Geometry check sheet. Reference: the model listing, model coordinates, mm. A direction names the side the tool comes from. Coordinates: 2 decimals unless noted, no trailing zeros. Loops run counter-clockwise (first coordinate to the right, second up) from the corner with the lowest first, then second, coordinate; pieces in that order, holes last. Notation, with made-up numbers: (77, 78) - (94, 78) arc R19 cw to (94, 82) - close; hole circle Ø7 at (33, 26). An arc over 180 degrees is marked (long way). Write item = value, one per line. Start each with the question number.
from build123d import *

# Parameters (mm, degrees)
SKETCH1_R           = 3.2639
BOSS_EXTRUDE1_DEPTH = 152.4


with BuildPart() as part:
    # Sketch1 → Boss-Extrude1 (new, symmetric)
    with BuildSketch(Plane.XY):
        with BuildLine():
            Line((-6.731, 4.575738531), (-6.731, -4.575738531))
            Line((-6.731, -4.575738531), (-12.442261469, -10.287))
            Line((-12.442261469, -10.287), (-15.6718, -10.287))
            Line((-15.6718, -10.287), (-15.6718, -6.858))
            Line((-15.6718, -6.858), (-14.478, -6.858))
            Line((-14.478, -6.858), (-14.478, -4.064))
            Line((-14.478, -4.064), (-19.05, -4.064))
            Line((-19.05, -4.064), (-19.05, -15.875))
            ThreePointArc((-19.05, -15.875), (-18.12006403, -18.12006403), (-15.875, -19.05))
            Line((-15.875, -19.05), (-4.064, -19.05))
            Line((-4.064, -19.05), (-4.064, -14.478))
            Line((-4.064, -14.478), (-6.858, -14.478))
            Line((-6.858, -14.478), (-6.858, -15.6718))
            Line((-6.858, -15.6718), (-10.287, -15.6718))
            Line((-10.287, -15.6718), (-10.287, -12.442261469))
            Line((-10.287, -12.442261469), (-4.575738531, -6.731))
            Line((-4.575738531, -6.731), (4.575738531, -6.731))
            Line((4.575738531, -6.731), (10.287, -12.442261469))
            Line((10.287, -12.442261469), (10.287, -15.6718))
            Line((10.287, -15.6718), (6.858, -15.6718))
            Line((6.858, -15.6718), (6.858, -14.478))
            Line((6.858, -14.478), (4.064, -14.478))
            Line((4.064, -14.478), (4.064, -19.05))
            Line((4.064, -19.05), (15.875, -19.05))
            ThreePointArc((15.875, -19.05), (18.12006403, -18.12006403), (19.05, -15.875))
            Line((19.05, -15.875), (19.05, -4.064))
            Line((19.05, -4.064), (14.478, -4.064))
            Line((14.478, -4.064), (14.478, -6.858))
            Line((14.478, -6.858), (15.6718, -6.858))
            Line((15.6718, -6.858), (15.6718, -10.287))
            Line((15.6718, -10.287), (12.442261469, -10.287))
            Line((12.442261469, -10.287), (6.731, -4.575738531))
            Line((6.731, -4.575738531), (6.731, 4.575738531))
            Line((6.731, 4.575738531), (12.442261469, 10.287))
            Line((12.442261469, 10.287), (15.6718, 10.287))
            Line((15.6718, 10.287), (15.6718, 6.858))
            Line((15.6718, 6.858), (14.478, 6.858))
            Line((14.478, 6.858), (14.478, 4.064))
            Line((14.478, 4.064), (19.05, 4.064))
            Line((19.05, 4.064), (19.05, 15.875))
            ThreePointArc((19.05, 15.875), (18.12006403, 18.12006403), (15.875, 19.05))
            Line((15.875, 19.05), (4.064, 19.05))
            Line((4.064, 19.05), (4.064, 14.478))
            Line((4.064, 14.478), (6.858, 14.478))
            Line((6.858, 14.478), (6.858, 15.6718))
            Line((6.858, 15.6718), (10.287, 15.6718))
            Line((10.287, 15.6718), (10.287, 12.442261469))
            Line((10.287, 12.442261469), (4.575738531, 6.731))
            Line((4.575738531, 6.731), (-4.575738531, 6.731))
            Line((-4.575738531, 6.731), (-10.287, 12.442261469))
            Line((-10.287, 12.442261469), (-10.287, 15.6718))
            Line((-10.287, 15.6718), (-6.858, 15.6718))
            Line((-6.858, 15.6718), (-6.858, 14.478))
            Line((-6.858, 14.478), (-4.064, 14.478))
            Line((-4.064, 14.478), (-4.064, 19.05))
            Line((-4.064, 19.05), (-15.875, 19.05))
            ThreePointArc((-15.875, 19.05), (-18.12006403, 18.12006403), (-19.05, 15.875))
            Line((-19.05, 15.875), (-19.05, 4.064))
            Line((-19.05, 4.064), (-14.478, 4.064))
            Line((-14.478, 4.064), (-14.478, 6.858))
            Line((-14.478, 6.858), (-15.6718, 6.858))
            Line((-15.6718, 6.858), (-15.6718, 10.287))
            Line((-15.6718, 10.287), (-12.442261469, 10.287))
            Line((-12.442261469, 10.287), (-6.731, 4.575738531))
        make_face()
        with Locations(Location((0, 0, 0), (0, 0, 180))):
            Circle(SKETCH1_R, mode=Mode.SUBTRACT)
        with BuildLine():
            Line((-11.8872, 17.272), (-14.478, 17.272))
            ThreePointArc((-14.478, 17.272), (-16.453656347, 16.453656347), (-17.272, 14.478))
            Line((-17.272, 14.478), (-17.272, 11.8872))
            Line((-17.272, 11.8872), (-11.8872, 11.8872))
            Line((-11.8872, 11.8872), (-11.8872, 17.272))
        make_face(mode=Mode.SUBTRACT)
        with BuildLine():
            Line((14.478, 17.272), (11.8872, 17.272))
            Line((11.8872, 17.272), (11.8872, 11.8872))
            Line((11.8872, 11.8872), (17.272, 11.8872))
            Line((17.272, 11.8872), (17.272, 14.478))
            ThreePointArc((17.272, 14.478), (16.453656347, 16.453656347), (14.478, 17.272))
        make_face(mode=Mode.SUBTRACT)
        with BuildLine():
            Line((11.8872, -17.272), (14.478, -17.272))
            ThreePointArc((14.478, -17.272), (16.453656347, -16.453656347), (17.272, -14.478))
            Line((17.272, -14.478), (17.272, -11.8872))
            Line((17.272, -11.8872), (11.8872, -11.8872))
            Line((11.8872, -11.8872), (11.8872, -17.272))
        make_face(mode=Mode.SUBTRACT)
        with BuildLine():
            Line((-14.478, -17.272), (-11.8872, -17.272))
            Line((-11.8872, -17.272), (-11.8872, -11.8872))
            Line((-11.8872, -11.8872), (-17.272, -11.8872))
            Line((-17.272, -11.8872), (-17.272, -14.478))
            ThreePointArc((-17.272, -14.478), (-16.453656347, -16.453656347), (-14.478, -17.272))
        make_face(mode=Mode.SUBTRACT)
    extrude(amount=BOSS_EXTRUDE1_DEPTH, both=True)


solid = part.part
(1) Tool access check on faces 4 (the face through (15, 11.887, -2)), 5 (the face through (-19.05, -10, 2)). Record the directions out of +Z, -Z, +X, -X, +Y, -Y that give a thin tool (end or side, any length) a straight path to the whole face; none if there is none.
(2) Scan lines: line 1 (Y direction, x = -14, z = -93); line 2 (X direction, y = -4.5, z = 135). Record each from-to range of solid material in increasing order.
(3) Sectioned sample at C-C on z = 43. Count the separate pieces of the cut face and the enclosed holes in it, plus the area to 3 significant figures.
(4) Depth check by flat-ended pin: pin 1 (1.4 mm diameter, centred on y = -18, z = 72, fed in from -X); pin 2 (7.5 mm diameter, centred on x = 0, z = 61.5, fed in from -Y); pin 3 (1.4 mm diameter, centred on y = 17, z = 65, fed in from -X). Enter the tip coordinate at first touch or a pass-through.
(5) Draft check along X on faces 1 (the face through (-3, 3, -152.4)), 2 (the face through (-19.05, 10, 2)), 3 (the face through (9.547, 7.391, 2.134)). Enter one of: pulls with the +X half, pulls with the -X half, needs draft (parallel to the pull), parting line crosses it, or undercut.
(6) Sectioned sample at A-A on x = 0. Enter the section's corners in (y, z).
Working result:
q1.face_4 = +Z, -Z
q1.face_5 = +Z, -Z, -X, +Y, -Y
q2.line_1 = -19.05 to -17.27, -11.89 to -10.29, 10.29 to 11.89, 17.27 to 19.05
q2.line_2 = -19.05 to -14.48, -6.73 to 6.73, 14.48 to 19.05
q3.separate_pieces = 1
q3.enclosed_holes = 5
q3.area = 612 mm2
q4.pin_1 = -18.71
q4.pin_2 = -6.73
q4.pin_3 = -19.02
q5.face_1 = needs draft
q5.face_2 = pulls with the -X half
q5.face_3 = undercut
q6.outline = (-6.73, -152.4) - (-3.26, -152.4) - (-3.26, 152.4) - (-6.73, 152.4) - close; (3.26, -152.4) - (6.73, -152.4) - (6.73, 152.4) - (3.26, 152.4) - close
